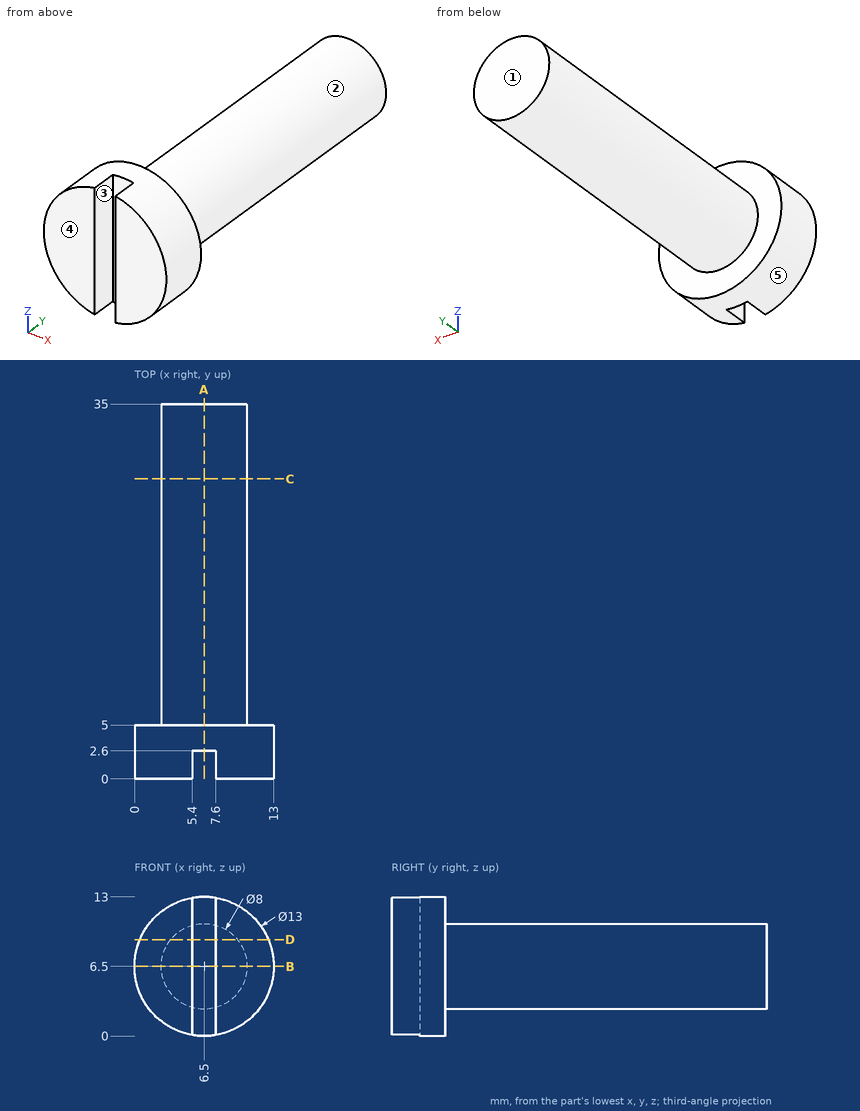
Verification items for this drawing (mm, ordinates from the low corner). A direction names the side the tool comes from. Give positions to 0.01 mm unless a question says otherwise; leave off trailing zeros. Order: outer loops, then holes, each group sorted by start corner. A loop starts at its lowest first (then second) coordinate and runs counter-clockwise, first axis right, second up. Notation, with made-up numbers: M 82.25,-20 L 130.25,-20 A29 ccw 130.25,17 Z; hole C 36.5,-12 d7. An arc over 180 degrees is marked long. Use a Markdown table: item, result.
Item 1: Depth check by flat-ended pin: P1, Ø1.5, axis at y = 30.5, z = 2.5, coming from the -X side; P2, Ø2, axis at x = 9, y = 20, coming from the -Z side; P3, Ø1.5, axis at x = 1.5, z = 11.5, coming from the +Y side. Enter the tip coordinate at first touch or a pass-through.
Answers follow:
| item | result |
|---|---|
| P1 | stops at x = 4.17 |
| P2 | stops at z = 2.79 |
| P3 | stops at y = 5 |
Item 2: Tool access check on the marked faces 1 and 2. Record the directions out of +Z, -Z, +X, -X, +Y, -Y that give a thin tool (end or side, any length) a straight path to the whole face; none if there is none.
Answers follow:
| item | result |
|---|---|
| face 1 | +Z, -Z, +X, -X, +Y |
| face 2 | +Y |
Item 3: Section check A-A (x = 6.5). Record the cut outline in (y, z).
Answers follow:
| item | result |
|---|---|
| outline | M 2.6,0 L 5,0 L 5,2.5 L 35,2.5 L 35,10.5 L 5,10.5 L 5,13 L 2.6,13 Z |
Item 4: Section check B-B (z = 6.5). Record the cut outline in (x, y).
Answers follow:
| item | result |
|---|---|
| outline | M 0,0 L 5.4,0 L 5.4,2.6 L 7.6,2.6 L 7.6,0 L 13,0 L 13,5 L 10.5,5 L 10.5,35 L 2.5,35 L 2.5,5 L 0,5 Z |
Item 5: Section check C-C (y = 28). Record the cut outline in (x, z), and give its area (3 significant figures).
Answers follow:
| item | result |
|---|---|
| outline | C 6.5,6.5 d8 |
| area | 50.3 mm2 |
Item 6: Material ranges on line 1 along Y through (x, z) = (1.5, 7.75); line 2 along X through (y, z) = (18, 6.25); line 3 along X through (y, z) = (1, 2.75), recorded low to high.
Answers follow:
| item | result |
|---|---|
| line 1 | y = 0 to 5 |
| line 2 | x = 2.51 to 10.49 |
| line 3 | x = 1.19 to 5.4, 7.6 to 11.81 |
Item 7: Section check D-D (z = 9). Record the cut outline in (x, y), and give its area (3 significant figures).
Answers follow:
| item | result |
|---|---|
| outline | M 0.5,0 L 5.4,0 L 5.4,2.6 L 7.6,2.6 L 7.6,0 L 12.5,0 L 12.5,5 L 9.62,5 L 9.62,35 L 3.38,35 L 3.38,5 L 0.5,5 Z |
| area | 242 mm2 |
Item 8: Draft check along X on the marked faces 3, 4 and 5. Enter one of: +X half, -X half, draft (parallel to the pull), parting line (faces both ways), or undercut.
Answers follow:
| item | result |
|---|---|
| face 3 | undercut |
| face 4 | draft |
| face 5 | parting line |
